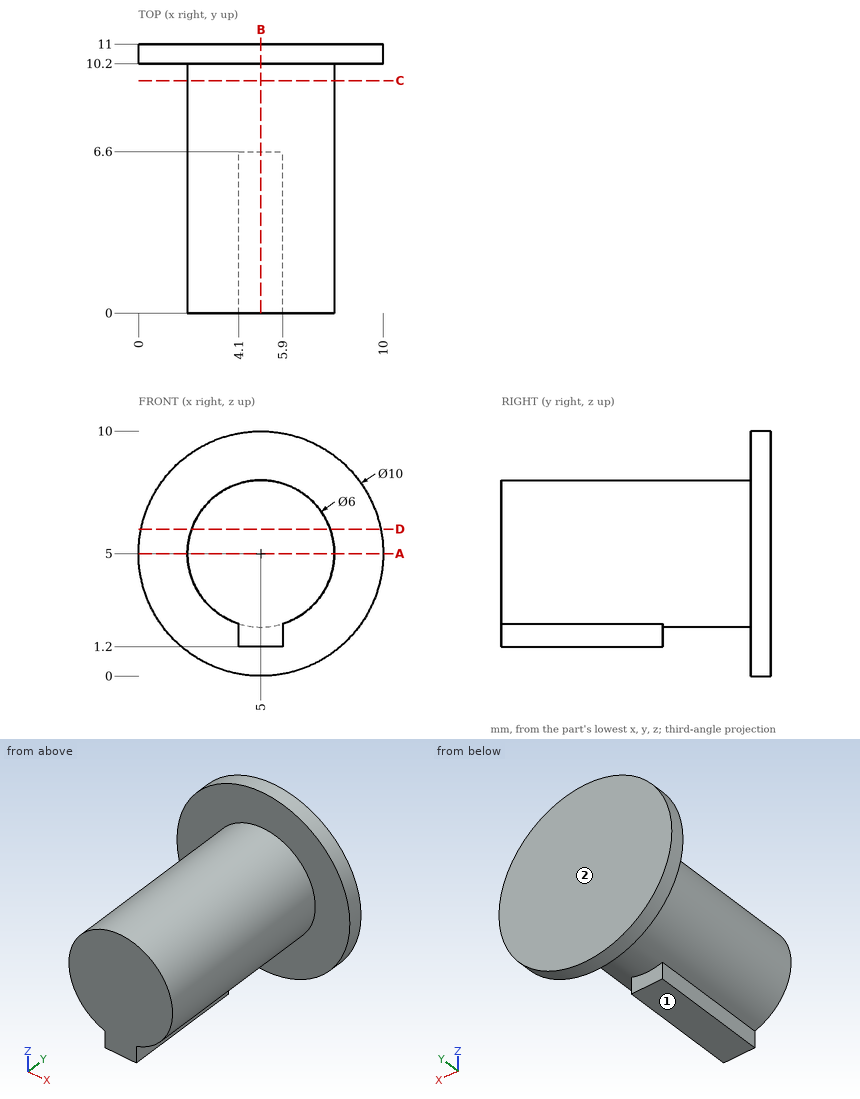
The drawing under review shows one solid part. Ordinate dimensions are in mm from its lowest x, y, z. A direction names the side the tool comes from. Coordinates: 2 decimals unless noted, no trailing zeros. Order: outer loops, then holes, each group sorted by start corner. A loop starts at its lowest first (then second) coordinate and runs counter-clockwise, first axis right, second up. Notation, with made-up numbers: M 33.5,59.5 L 42.5,59.5 A23 ccw 42.5,94.5 Z; hole C 28,49.5 d7. An arc over 180 degrees is marked long. One line per question, with ' | ' between items.
(1) Add section C-C, the plane y = 9.5. Write out the cut boundary in (x, z).
Geometry results:
outline: C 5,5 d6
(2) Add section D-D, the plane z = 6. Write out the cut boundary in (x, y), then the cut area to 3 significant figures.
Geometry results:
outline: M 0.1,10.2 L 2.17,10.2 L 2.17,0 L 7.83,0 L 7.83,10.2 L 9.9,10.2 L 9.9,11 L 0.1,11 Z | area: 65.5 mm²
(3) Machinability: for the marked faces 1 and 2, which of the approach directions +Z, -Z, +X, -X, +Y, -Y give a long, thin tool a straight path to every point of the face, cutting with its end or side? Answer none if there is none.
Geometry results:
face 1: -Z, +X, -X, -Y | face 2: +Z, -Z, +X, -X, +Y
(4) Insertion check: pin 1 (2 mm diameter, centred on x = 2.5, y = 4.5, fed in from +Z); pin 2 (0.5 mm diameter, centred on x = 4.5, y = 4, fed in from -Z); pin 3 (0.5 mm diameter, centred on y = 3.5, z = 1.5, fed in from +X). Each pin has a flat end and moves straight along its axis. Give the tip position at first contact, or say it passes through.
Geometry results:
pin 1: stops at z = 7.6 | pin 2: stops at z = 1.2 | pin 3: stops at x = 5.9
(5) Add section A-A, the plane z = 5. Write out the cut boundary in (x, y).
Geometry results:
outline: M 0,10.2 L 2,10.2 L 2,0 L 8,0 L 8,10.2 L 10,10.2 L 10,11 L 0,11 Z
(6) Add section B-B, the plane x = 5. Write out the cut boundary in (y, z).
Geometry results:
outline: M 0,1.2 L 6.6,1.2 L 6.6,2 L 10.2,2 L 10.2,0 L 11,0 L 11,10 L 10.2,10 L 10.2,8 L 0,8 Z
(7) For probe 1 along Y at (x, z) = (2.5, 7.75); probe 2 along X at (y, z) = (9.5, 5); probe 3 along Z at (x, y) = (5, 0.5), list the stretches that pass through material, from the lowest coordinate up. Write a range as from..to.
Geometry results:
probe 1: y = 10.2..11 | probe 2: x = 2..8 | probe 3: z = 1.2..8
